Geometry: final body of the model. Coordinates: model frame, mm. A direction names the side the tool comes from. Give positions to 0.01 mm unless a question says otherwise; leave off trailing zeros. Loops run counter-clockwise (first coordinate to the right, second up) from the corner with the lowest first, then second, coordinate; pieces in that order, holes last.
from build123d import *

# Parameters (mm, degrees)
SKETCH1_R           = 1.4
BOSS_EXTRUDE1_DEPTH = 0.8
SKETCH2_R           = 0.6
SKETCH2_R_2         = 0.2
CUT_EXTRUDE1_DEPTH  = 0.8
SKETCH3_R           = 2.5
SKETCH3_R_2         = 1.5
SKETCH3_R_3         = 0.2
BOSS_EXTRUDE2_DEPTH = 0.0254
SKETCH4_R           = 0.6
SKETCH4_R_2         = 0.2
BOSS_EXTRUDE3_DEPTH = 0.0254


with BuildPart() as part:
    # Sketch1 → Boss-Extrude1 (new body)
    with BuildSketch(Plane(origin=(0, 0, 0), x_dir=(1, 0, 0), z_dir=(0, 1, 0))):
        with BuildLine():
            Line((-2.6, 0), (-2.6, 1.51002008))
            ThreePointArc((-2.6, 1.51002008), (0, 7.6), (2.6, 1.51002008))
            Line((2.6, 1.51002008), (2.6, 0))
            ThreePointArc((2.6, 0), (0, -2.6), (-2.6, 0))
        make_face()
        with Locations(Location((0, 4, 0), (0, 0, 270))):
            Circle(SKETCH1_R, mode=Mode.SUBTRACT)
    extrude(amount=BOSS_EXTRUDE1_DEPTH)

    # Sketch2 → Cut-Extrude1 (cut)
    with BuildSketch(Plane(origin=(0, 0.8, 0), x_dir=(1, 0, 0), z_dir=(0, 1, 0))):
        with Locations(Location((0, 0, 0), (0, 0, 270))):
            Circle(SKETCH2_R)
        with Locations(Location((-1.5, 1.4, 0), (0, 0, 270))):
            Circle(SKETCH2_R_2)
    extrude(amount=-CUT_EXTRUDE1_DEPTH, mode=Mode.SUBTRACT)

    # Sketch3 → Boss-Extrude2 (add)
    with BuildSketch(Plane(origin=(0, 0.8, 0), x_dir=(1, 0, 0), z_dir=(0, 1, 0))):
        with Locations(Location((0, 0, 0), (0, 0, 270))):
            Circle(SKETCH3_R)
        with Locations(Location((0, 0, 0), (0, 0, 270))):
            Circle(SKETCH3_R_2, mode=Mode.SUBTRACT)
        with Locations(Location((-1.5, 1.4, 0), (0, 0, 270))):
            Circle(SKETCH3_R_3, mode=Mode.SUBTRACT)
    extrude(amount=BOSS_EXTRUDE2_DEPTH)

    # Sketch4 → Boss-Extrude3 (add)
    with BuildSketch(Plane.XZ):
        with BuildLine():
            ThreePointArc((-1.270694255, -1.797463292), (-1.103147311, -1.172970136), (-1.727640466, -1.005423192))
            ThreePointArc((-1.727640466, -1.005423192), (0.511420208, -7.419163817), (0.775806401, -0.63097102))
            ThreePointArc((0.775806401, -0.63097102), (-0.211741678, 0.977325668), (-0.445093544, -0.89548408))
            ThreePointArc((-0.445093544, -0.89548408), (-0.358340982, -1.283942918), (0, -1.4572))
            ThreePointArc((0, -1.4572), (0.657731518, -6.456261609), (-1.270694255, -1.797463292))
        make_face()
        with Locations(Location((0, 0, 0), (0, 0, 90))):
            Circle(SKETCH4_R, mode=Mode.SUBTRACT)
        with Locations(Location((-1.5, -1.4, 0), (0, 0, 90))):
            Circle(SKETCH4_R_2, mode=Mode.SUBTRACT)
    extrude(amount=BOSS_EXTRUDE3_DEPTH)


solid = part.part
Item 1: Section query A-A on y = 0.65. Return loops of the section in (x, z).
Values follow:
outline: (-2.6, -1.51) arc R3.6 ccw (long way) to (2.6, -1.51) - (2.6, 0) arc R2.6 ccw to (-2.6, 0) - close; hole circle Ø0.4 at (-1.5, -1.4); hole circle Ø2.8 at (0, -4); hole circle Ø1.2 at (0, 0)
Item 2: Pin query (flat end, axial travel): pin 1 (3.5 mm diameter, centred on x = 0, z = -1, fed in from +Y); pin 2 (3 mm diameter, centred on x = 0, z = -4, fed in from -Y). Return the tip coordinate at first contact, or that it passes through.
Values follow:
pin 1: stops at y = 0.83
pin 2: stops at y = 0
Item 3: Ray query, probe 1 along X at (y, z) = (0.6, -1.4); probe 2 along Y at (x, z) = (2.25, -2); probe 3 along Z at (x, y) = (-0.25, 0.55). Return the intervals inside material, ascending.
Values follow:
probe 1: x = -2.6 to -1.7, -1.3 to 2.6
probe 2: y = -0.03 to 0.8
probe 3: z = -7.59 to -5.38, -2.62 to -0.55, 0.55 to 2.59
Item 4: Draft query along X for faces 1 (the face through (2, 0.8, -4)), 2 (the face through (-0.1, 0.4, -7.6)), 3 (the face through (-1, 0, -1)). Return one class per face: +X half, -X half, draft (parallel to the pull), parting line (faces both ways), or undercut.
Values follow:
face 1: draft
face 2: parting line
face 3: undercut
Item 5: Set-up query: faces 4 (the face through (0.421, 0.394, -2.665)), 5 (the face through (-1, 0.8, 0)). Return all of +Z, -Z, +X, -X, +Y, -Y with unobstructed straight access to the full face (end or side cutting, diameter ignored); none if empty.
Values follow:
face 4: +Y, -Y
face 5: +Y
